For this review, take the finished solid that the model builds, in its own axes (mm). A direction names the side the tool comes from. Give positions to 0.01 mm unless a question says otherwise; leave off trailing zeros. Order: outer loops, then holes, each group sorted by start corner. A loop starts at its lowest first (then second) coordinate and runs counter-clockwise, first axis right, second up. Notation, with made-up numbers: (19, 39) -> (45, 39) arc R22 ccw to (45, 61) -> close; hole circle Ø4 at (55.5, 34). An arc over 180 degrees is marked (long way). Return JSON: item names as keys, results as strings. Group by question number.
1) The part is to be moulded in two halves that separate along X. For faces 4 (the face through (-17.718, 11.657, 16.731)), 5 (the face through (-19.1, 13.1, 17.2)), 6 (the face through (4, -27.636, 17)), say which applies: released by +X, released by -X, zero draft, split by the parting line, or undercut.
2) Add section A-A (z = 16.5). Give the boundary of the cut face in (x, y).
3) To check wall thickness, follow line 1 along X through (y, z) = (-12, 3.5); line 2 along Y through (x, z) = (9.5, 11); line 3 along X through (y, z) = (-7.5, 32). State the ranges of each line that lie inside material, in increasing order.
4) Insertion check: P1, Ø0.8, axis at x = 4, y = -26.5, coming from the -Z side; P2, Ø1.5, axis at x = 3, y = -3, coming from the -Z side; P3, Ø1.6, axis at x = 5.5, y = -26.5, coming from the +Z side; P4, Ø5, axis at x = 20.5, y = -15, coming from the -Z side. Each pin has a flat end and moves straight along its axis. Give the tip position at first contact, or say it passes through.
5) Add section B-B (x = 4). State how many separate pieces and enclosed holes the cut face has, then the cut area to 3 significant figures.
6) For faces 1 (the face through (-1, -25, 28)), 2 (the face through (4, -26, 35)), 3 (the face through (4, -26, 5)), list the 3-axis set-ups (+Z, -Z, +X, -X, +Y, -Y) from which the entire face can be reached by the end or side of a thin tool; tool diameter is ignored.
from build123d import *

# Parameters (mm, degrees)
SKETCH_1_W          = 55
SKETCH_1_H          = 45
EXTRUDE_1_DEPTH     = 35
SKETCH_4_R          = 20.5
EXTRUDE_3_DEPTH     = 2
FILLET_2_R          = 15
FILLET_3_R          = 15
FILLET_4_R          = 1
SHELL_1_T           = -2
EXTRUDE_START       = 5
SKETCH_7_R          = 21.5
SKETCH_7_R_2        = 20.5
EXTRUDE_4_DEPTH     = 5
FILLET_5_R          = 1
FILLET_6_R          = 0.5
CUT_EXTRUDE_1_REACH = 73.818
SKETCH_8_W          = 5
SKETCH_8_H          = 10
CUT_EXTRUDE_2_REACH = 68.168
SKETCH_14_W         = 15
SKETCH_14_H         = 3
CUT_EXTRUDE_3_REACH = 68.168
SKETCH_17_W         = 15
SKETCH_17_H         = 3
FILLET_9_R          = 0.5


with BuildPart() as part:
    # 스케치1 → 보스-돌출1 (new body)
    with BuildSketch(Plane.XY):
        with Locations((3.872936318, -5.136103152)):
            Rectangle(SKETCH_1_W, SKETCH_1_H)
    extrude(amount=EXTRUDE_1_DEPTH)

    # 스케치4 → 보스-돌출3 (add)
    with BuildSketch(Plane(origin=(-2.164184789, -3.486971785, 35), x_dir=(1, 0, 0), z_dir=(0, 0, 1))):
        with Locations((6.037121107, -1.171687144)):
            Circle(SKETCH_4_R)
    extrude(amount=EXTRUDE_3_DEPTH)

    # 필렛2
    fillet_2_edges = [part.edges().sort_by_distance(p)[0] for p in [
        (31.372936318, 17.363896848, 17.5),
    ]]
    fillet(fillet_2_edges, radius=FILLET_2_R)

    # 필렛3
    fillet_3_edges = [part.edges().sort_by_distance(p)[0] for p in [
        (-23.627063682, 17.363896848, 17.5),
        (31.372936318, -27.636103152, 17.5),
        (-23.627063682, -27.636103152, 17.5),
    ]]
    fillet(fillet_3_edges, radius=FILLET_3_R)

    # 필렛4
    fillet_4_edges = [part.edges().sort_by_distance(p)[0] for p in [
        (3.872936318, 17.363896848, 35),
        (26.979538036, 12.970498566, 35),
        (3.872936318, -27.636103152, 35),
        (-23.627063682, -5.136103152, 35),
        (31.372936318, -5.136103152, 35),
        (-19.2336654, 12.970498566, 35),
        (26.979538036, -23.24270487, 35),
        (-19.2336654, -23.24270487, 35),
    ]]
    fillet(fillet_4_edges, radius=FILLET_4_R)

    # 쉘1
    shell_1_openings = [part.faces().sort_by_distance(p)[0] for p in [
        (3.872936318, -5.136103152, 0),
    ]]
    offset(amount=SHELL_1_T, openings=shell_1_openings, kind=Kind.INTERSECTION)

    # 스케치7 → 보스-돌출4 (add)
    with BuildSketch(Plane(origin=(0, 0, 33), x_dir=(-1, 0, 0), z_dir=(0, 0, -1)).offset(EXTRUDE_START)):
        with Locations((-3.872936318, -4.658658928)):
            Circle(SKETCH_7_R)
        with Locations(Location((-3.872936318, -4.658658928, 0), (0, 0, 180))):
            Circle(SKETCH_7_R_2, mode=Mode.SUBTRACT)
    extrude(amount=-EXTRUDE_4_DEPTH)

    # 필렛5
    fillet_5_edges = [part.edges().sort_by_distance(p)[0] for p in [
        (-16.627063682, -4.658658928, 37),
    ]]
    fillet(fillet_5_edges, radius=FILLET_5_R)

    # 필렛6
    fillet_6_edges = [part.edges().sort_by_distance(p)[0] for p in [
        (-16.627063682, -4.658658928, 35),
    ]]
    fillet(fillet_6_edges, radius=FILLET_6_R)

    # 스케치8 → 컷-돌출1 (cut, up to next)
    with BuildSketch(Plane(origin=(31.372936318, 0, 0), x_dir=(0, 0, -1), z_dir=(1, 0, 0)), mode=Mode.PRIVATE) as cut_extrude_1_sk1:
        with Locations((-5.5, -5.136103152)):
            Rectangle(SKETCH_8_W, SKETCH_8_H)
    cut_extrude_1_tool1 = extrude(cut_extrude_1_sk1.sketch, amount=-CUT_EXTRUDE_1_REACH, mode=Mode.PRIVATE) & part.part
    add(cut_extrude_1_tool1.solids().sort_by_distance((31.372936, -5.136103, 5.5))[0], mode=Mode.SUBTRACT)

    # 스케치14 → 컷-돌출2 (cut, up to next)
    with BuildSketch(Plane(origin=(0, 17.363896848, 0), x_dir=(1, 0, 0), z_dir=(0, 1, 0)), mode=Mode.PRIVATE) as cut_extrude_2_sk1:
        with Locations((3.872936318, -3.5)):
            Rectangle(SKETCH_14_W, SKETCH_14_H)
    cut_extrude_2_tool1 = extrude(cut_extrude_2_sk1.sketch, amount=-CUT_EXTRUDE_2_REACH, mode=Mode.PRIVATE) & part.part
    add(cut_extrude_2_tool1.solids().sort_by_distance((3.872936, 17.363897, 3.5))[0], mode=Mode.SUBTRACT)

    # 스케치17 → 컷-돌출3 (cut, up to next)
    with BuildSketch(Plane.XZ.offset(27.636103152), mode=Mode.PRIVATE) as cut_extrude_3_sk1:
        with Locations((3.872936318, 3.5)):
            Rectangle(SKETCH_17_W, SKETCH_17_H)
    cut_extrude_3_tool1 = extrude(cut_extrude_3_sk1.sketch, amount=-CUT_EXTRUDE_3_REACH, mode=Mode.PRIVATE) & part.part
    add(cut_extrude_3_tool1.solids().sort_by_distance((3.872936, -27.636103, 3.5))[0], mode=Mode.SUBTRACT)

    # 필렛9
    fillet_9_edges = [part.edges().sort_by_distance(p)[0] for p in [
        (31.372936318, -5.136103152, 3),
        (31.372936318, -0.136103152, 5.5),
        (31.372936318, -5.136103152, 8),
        (31.372936318, -10.136103152, 5.5),
        (11.372936318, 15.363896848, 3.5),
        (3.872936318, 15.363896848, 2),
        (-3.627063682, 17.363896848, 3.5),
        (3.872936318, 17.363896848, 5),
        (3.872936318, -27.636103152, 5),
        (11.372936318, -27.636103152, 3.5),
        (3.872936318, -27.636103152, 2),
        (-3.627063682, -27.636103152, 3.5),
    ]]
    fillet(fillet_9_edges, radius=FILLET_9_R)


solid = part.part
Evaluation:
{
 "1": {"face 4": "undercut", "face 5": "released by -X", "face 6": "zero draft"},
 "2": {"outline": "(-23.63, -12.64) arc R15 ccw to (-8.63, -27.64) -> (16.37, -27.64) arc R15 ccw to (31.37, -12.64) -> (31.37, 2.36) arc R15 ccw to (16.37, 17.36) -> (-8.63, 17.36) arc R15 ccw to (-23.63, 2.36) -> close; hole (-21.63, -12.64) arc R13 ccw to (-8.63, -25.64) -> (16.37, -25.64) arc R13 ccw to (29.37, -12.64) -> (29.37, 2.36) arc R13 ccw to (16.37, 15.36) -> (-8.63, 15.36) arc R13 ccw to (-21.63, 2.36) -> close"},
 "3": {"line 1": "-23.63 to -21.63, 29.37 to 31.37", "line 2": "-27.64 to -25.64, 15.36 to 17.36", "line 3": "-23.63 to -21.63, -17.44 to -16.43, 24.18 to 25.18, 29.37 to 31.37"},
 "4": {"P1": "z = 0", "P2": "z = 35", "P3": "z = 35", "P4": "z = 28"},
 "5": {"separate pieces": "3", "enclosed holes": "0", "area": "219 mm^2"},
 "6": {"face 1": "-Z", "face 2": "+Z", "face 3": "+Y, -Y"}
}
